Could you check a few things on this model? Use its own coordinates, in mm. Coordinates: 2 decimals unless noted, no trailing zeros. Write each loop counter-clockwise with the first axis right and the second up, starting at its lowest first coordinate (ties: lowest second). Pieces come first, ordered by that corner, then holes. Notation, with made-up numbers: (85, 62.25) - (93, 62.25) arc R35 cw to (93, 99.25) - close; hole circle Ø3 at (-32, 87). An arc over 180 degrees is marked (long way). Answer as a JSON object with one key per item and string values. Group by question number.
1) Will these pins go through, and if not, where does the flat tip stop? pin 1 Ø1.5 at (x, z) = (71.5, 1) entering from +Y; pin 2 Ø2.5 at (x, y) = (75.23, -38) entering from -Z.
2) If we section it at B-B (x = 11): Write out the boundary of the cut face in (y, z).
3) If we section it at D-D (y = -11): Write out the boundary of the cut face in (x, z).
4) Please list where these lines run through material, in increasing order: line 1 along X through (y, z) = (-38, 0.1); line 2 along X through (y, z) = (-7, 0.8); line 3 along X through (y, z) = (-26.5, 1.5).
5) If we section it at A-A (y = -43.38): Write out the boundary of the cut face in (x, z), plus the area to 3 significant figures.
6) If we section it at C-C (z = 1.4): State how many separate pieces and enclosed holes the cut face has, plus the area to 3 significant figures.
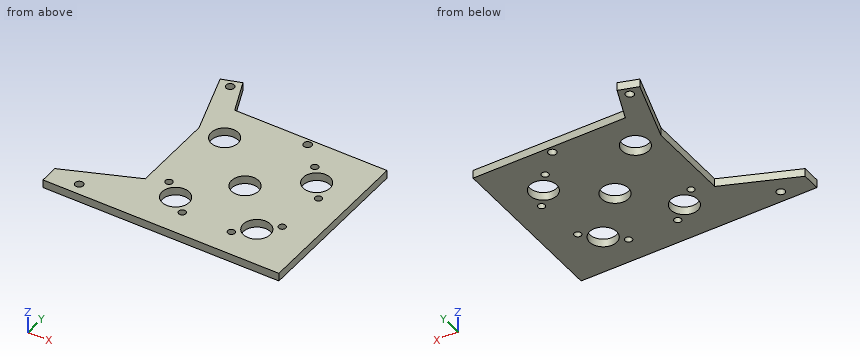
Autodesk Inventor part; units mm, degrees
ref_plane "YZ Plane" through (0, 0, 0) normal (1, 0, 0) x (0, 1, 0)
ref_plane "XZ Plane" through (0, 0, 0) normal (0, 1, 0) x (-1, 0, 0)
ref_plane "XY Plane" through (0, 0, 0) normal (0, 0, 1) x (1, 0, 0)
sketch "ギア線図" plane through (0, 0, 0) normal (0, 0, 1) x (1, 0, 0)
  circle A0 centre (11.2246, -29.111) radius 11.1
  circle A1 centre (54.3074, -26.8895) radius 20.05
  circle A2 centre (54.3074, -26.8895) radius 4.55
  circle A3 centre (35.8191, -9.9133) radius 11.1
  circle A4 centre (39.3074, -43.38) radius 2.05
  circle A5 centre (69.3074, -43.38) radius 2.05
  circle A6 centre (72.141, -13.5141) radius 2.05
  circle A7 centre (39.3074, -43.38) radius 15
  circle A8 centre (69.3074, -43.38) radius 15
  circle A9 centre (72.141, -13.5141) radius 15
  circle A10 centre (54.3074, -26.8895) radius 5.5 construction
  circle A11 centre (11.2246, -29.111) radius 13 construction
  circle A12 centre (54.3074, -26.8895) radius 20.5 construction
  circle A13 centre (35.8191, -9.9133) radius 20.55
  circle A14 centre (35.8191, -9.9133) radius 21.5 construction
  circle A15 centre (35.8191, -9.9133) radius 13 construction
  circle A16 centre (39.3074, -43.38) radius 2.5 construction
  circle A17 centre (69.3074, -43.38) radius 2.5 construction
  circle A18 centre (72.141, -13.5141) radius 2.5 construction
  circle A19 centre (11.2246, -29.111) radius 20.1
  circle A20 centre (11.2246, -29.111) radius 22 construction
  line L0 (39.3074, -43.38) -> (69.3074, -43.38)
  circle A21 centre (0, 0) radius 20.1
  circle A22 centre (0, 0) radius 22 construction
  circle A23 centre (39.3074, -43.38) radius 9.5 construction
  circle A24 centre (69.3074, -43.38) radius 9.5 construction
  circle A25 centre (72.141, -13.5141) radius 9.5 construction
  point P0 (58.2233, -20.0465)
  point P1 (42.0436, -35)
  point P2 (21.5995, 15.2696)
  point P3 (38.2329, 5.9161)
  point P4 (24.1755, 8.4229)
  point P5 (21.6039, 15.1272)
  point P6 (23.3458, 16.3469)
  point P7 (23.3177, 16.3886)
  dimension "d7" = 22.2
  dimension "d8" = 40.1
  dimension "d9" = 9.1
  dimension "d11" = 22.2
  dimension "d12" = 4.1
  dimension "d13" = 4.1
  dimension "d14" = 4.1
  dimension "d15" = 30
  dimension "d16" = 30
  dimension "d17" = 30
  dimension "d18" = 11
  dimension "d21" = 26
  dimension "d29" = 41
  dimension "d39" = 22.2921
  dimension "d40" = 22.2921
  dimension "d41" = 22.2921
  dimension "d43" = 41.1
  dimension "d44" = 43
  dimension "d45" = 26
  dimension "d46" = 5
  dimension "d47" = 5
  dimension "d48" = 5
  dimension "d49" = 40.2
  dimension "d50" = 44
  dimension "d53" = 40.2
  dimension "d55" = 44
  dimension "d58" = 19
  dimension "d59" = 19
  dimension "d60" = 19
sketch "スケッチ3" plane through (0, 0, 0) normal (0, 0, 1) x (1, 0, 0)
  circle A0 centre (54.3074, -26.8895) radius 20.05 construction
  circle A1 centre (39.3074, -43.38) radius 2.05 construction
  circle A2 centre (69.3074, -43.38) radius 2.05 construction
  circle A3 centre (72.141, -13.5141) radius 2.05 construction
  circle A4 centre (39.3074, -43.38) radius 15 construction
  circle A5 centre (69.3074, -43.38) radius 15 construction
  circle A6 centre (72.141, -13.5141) radius 15 construction
  line L0 (39.3074, -43.38) -> (45.2254, -48.7631)
  line L1 (45.2254, -48.7631) -> (39.3074, -43.38)
  line L2 (39.3074, -43.38) -> (33.3894, -37.9969)
  line L3 (39.3074, -43.38) -> (40.8161, -41.7214)
  circle A7 centre (33.3894, -37.9969) radius 1.3
  circle A8 centre (45.2254, -48.7631) radius 1.3
  line L4 (69.3074, -43.38) -> (67.7987, -41.7214)
  line L5 (69.3074, -43.38) -> (75.2254, -37.9969)
  line L6 (69.3074, -43.38) -> (63.3894, -48.7631)
  circle A9 centre (63.3894, -48.7631) radius 1.3
  circle A10 centre (75.2254, -37.9969) radius 1.3
  line L7 (72.141, -13.5141) -> (70.3474, -14.8594)
  line L8 (67.341, -7.1142) -> (72.141, -13.5141)
  line L9 (72.141, -13.5141) -> (76.9411, -19.9141)
  circle A11 centre (67.341, -7.1142) radius 1.3
  circle A12 centre (76.9411, -19.9141) radius 1.3
  circle A13 centre (39.3074, -43.38) radius 5
  circle A14 centre (69.3074, -43.38) radius 5
  circle A15 centre (72.141, -13.5141) radius 5
  circle A16 centre (54.3074, -26.8895) radius 5
  circle A17 centre (35.8191, -9.9133) radius 11.1 construction
  line L10 (87.141, -58.38) -> (21.087, -58.38)
  line L11 (87.141, 3.5148) -> (87.141, -58.38)
  circle A18 centre (35.8191, -9.9133) radius 5
  circle A19 centre (23.1948, 12.8161) radius 1.5
  circle A20 centre (59.3303, 1.1874) radius 1.5
  circle A21 centre (11.2246, -29.111) radius 5
  circle A22 centre (10.6068, -54.0855) radius 1.5
  line L12 (87.141, 3.5148) -> (30.8773, 3.5148)
  line L13 (30.8773, 3.5148) -> (25.4959, 16.5655)
  line L14 (26.368, -40.6885) -> (0, -51.5612)
  line L15 (0, -51.5612) -> (0, -58.38)
  line L16 (0, -58.38) -> (21.087, -58.38)
  line L17 (26.368, -40.6885) -> (26.368, -9.9133)
  line L18 (26.368, -9.9133) -> (18.5366, 14.3161)
  line L19 (18.5366, 14.3161) -> (25.4959, 16.5655)
  point P0 (0, 0)
  point P1 (0, 0)
  dimension "d61" = 8
  dimension "d62" = 8
  dimension "d63" = 2.6
  dimension "d64" = 2.6
  dimension "d65" = 8
  dimension "d66" = 8
  dimension "d67" = 2.6
  dimension "d68" = 2.6
  dimension "d69" = 8
  dimension "d70" = 8
  dimension "d71" = 2.6
  dimension "d72" = 2.6
  dimension "d73" = 10
  dimension "d74" = 10
  dimension "d75" = 10
  dimension "d76" = 10
  dimension "d79" = 10
extrude "押し出し1" add sketch "スケッチ3" along normal blind 3 contours L10 L16 L15 L14 L17 L18 L19 L13 L12 L11
sketch "スケッチ5" plane through (0, 0, 3) normal (0, 0, 1) x (1, 0, 0)
  circle A0 centre (10.6068, -54.0855) radius 1.5
  circle A1 centre (23.1948, 12.8161) radius 1.5
  circle A2 centre (59.3303, 1.1874) radius 1.5
  circle A3 centre (54.3074, -26.8895) radius 5
  circle A4 centre (35.8191, -9.9133) radius 5
  point P0 (0, 0)
equation "\"d40\" = d39"
equation "\"d41\" = d40"
properties part number "モーターマウント" material "アルミニウム 2014-T4"
Here are the results:
{
 "1": {"pin 1": "stops at y = 3.51", "pin 2": "passes through"},
 "2": {"outline": "(-58.38, 0) - (-55.53, 0) - (-55.53, 3) - (-58.38, 3) - close; (-52.64, 0) - (-47.03, 0) - (-47.03, 3) - (-52.64, 3) - close"},
 "3": {"outline": "(26.37, 0) - (30.94, 0) - (30.94, 3) - (26.37, 3) - close; (40.7, 0) - (67.82, 0) - (67.82, 3) - (40.7, 3) - close; (76.46, 0) - (87.14, 0) - (87.14, 3) - (76.46, 3) - close"},
 "4": {"line 1": "x = 26.37 to 32.09, 34.69 to 73.93, 76.53 to 87.14", "line 2": "x = 25.43 to 31.76, 39.88 to 66.05, 68.64 to 87.14", "line 3": "x = 26.37 to 49.32, 59.29 to 87.14"},
 "5": {"outline": "(19.84, 0) - (34.31, 0) - (34.31, 3) - (19.84, 3) - close; (44.31, 0) - (64.31, 0) - (64.31, 3) - (44.31, 3) - close; (74.31, 0) - (87.14, 0) - (87.14, 3) - (74.31, 3) - close", "area": "142 mm²"},
 "6": {"separate pieces": "1", "enclosed holes": "14", "area": "3,770 mm²"}
}
